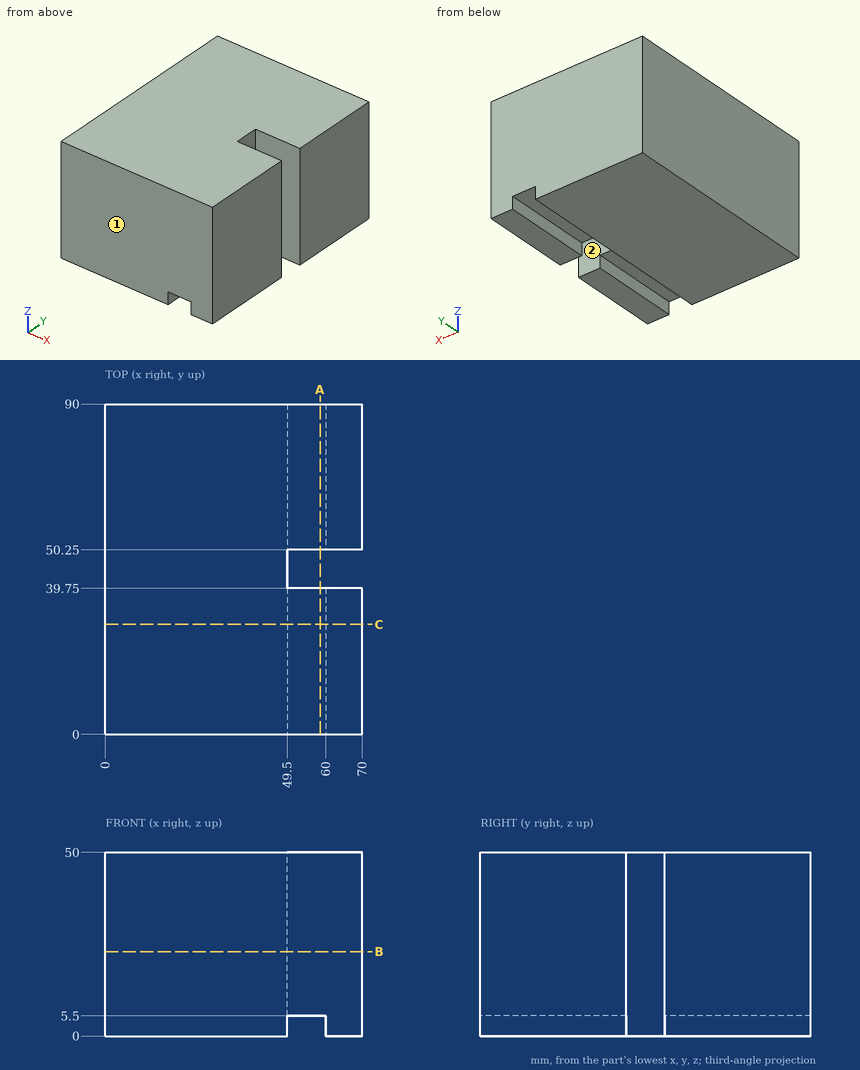
The figure shows three views and two pictorial views of one solid part (mm, origin at its lowest corner). Answer the questions. A direction names the side the tool comes from. Give positions to 0.01 mm unless a question says otherwise; leave off trailing zeros. Loops run counter-clockwise (first coordinate to the right, second up) from the corner with the lowest first, then second, coordinate; pieces in that order, holes last. Notation, with made-up numbers: (64, 31.25) -> (70, 31.25) arc R10 ccw to (70, 45.25) -> close; hole circle Ø5 at (15.5, -23.75). An arc over 180 degrees is marked (long way). Use CSV: the item, a comma, the result in double quotes.
1. The part is cut by section C-C (y = 30). Write down the section's boundary in (x, z).
Found:
outline,"(0, 0) -> (49.5, 0) -> (49.5, 5.5) -> (60, 5.5) -> (60, 0) -> (70, 0) -> (70, 50) -> (0, 50) -> close"
2. A tool of negligible diameter and unlimited length cuts with its end or side. For the marked faces 1 and 2, from which of +Z, -Z, +X, -X, +Y, -Y can it reach the whole face along a straight path? Write none if from no direction.
Found:
face 1,"+Z, -Z, +X, -X, -Y"
face 2,"+Z, -Z, +X"
3. The part is cut by section A-A (x = 58.5). Write down the section's boundary in (y, z).
Found:
outline,"(0, 5.5) -> (39.75, 5.5) -> (39.75, 50) -> (0, 50) -> close; (50.25, 5.5) -> (90, 5.5) -> (90, 50) -> (50.25, 50) -> close"
4. The part is cut by section B-B (z = 23). Write down the section's boundary in (x, y), then the cut area to 3 significant figures.
Found:
outline,"(0, 0) -> (70, 0) -> (70, 39.75) -> (49.5, 39.75) -> (49.5, 50.25) -> (70, 50.25) -> (70, 90) -> (0, 90) -> close"
area,"6,080 mm^2"
5. Straight lines are drawn through the part: line 1 (Y direction, x = 62.5, z = 40); line 2 (X direction, y = 43.5, z = 30.5); line 3 (Z direction, x = 52, y = 55). For each, find the intervals that lie inside material, in ascending order.
Found:
line 1,"0 to 39.75, 50.25 to 90"
line 2,"0 to 49.5"
line 3,"5.5 to 50"
